Design review of the part shown in the three views and the two pictorial views. Dimensions are in mm from the part's minimum x, y and z. Coordinates: 2 decimals unless noted, no trailing zeros. Loops run counter-clockwise (first coordinate to the right, second up) from the corner with the lowest first, then second, coordinate; pieces in that order, holes last. Notation, with made-up numbers: M 65,59 L 103,59 A21 ccw 103,66 Z; hole C -9.5,-18.75 d9. An arc over 180 degrees is marked long. Use one line per item in the form item = value.
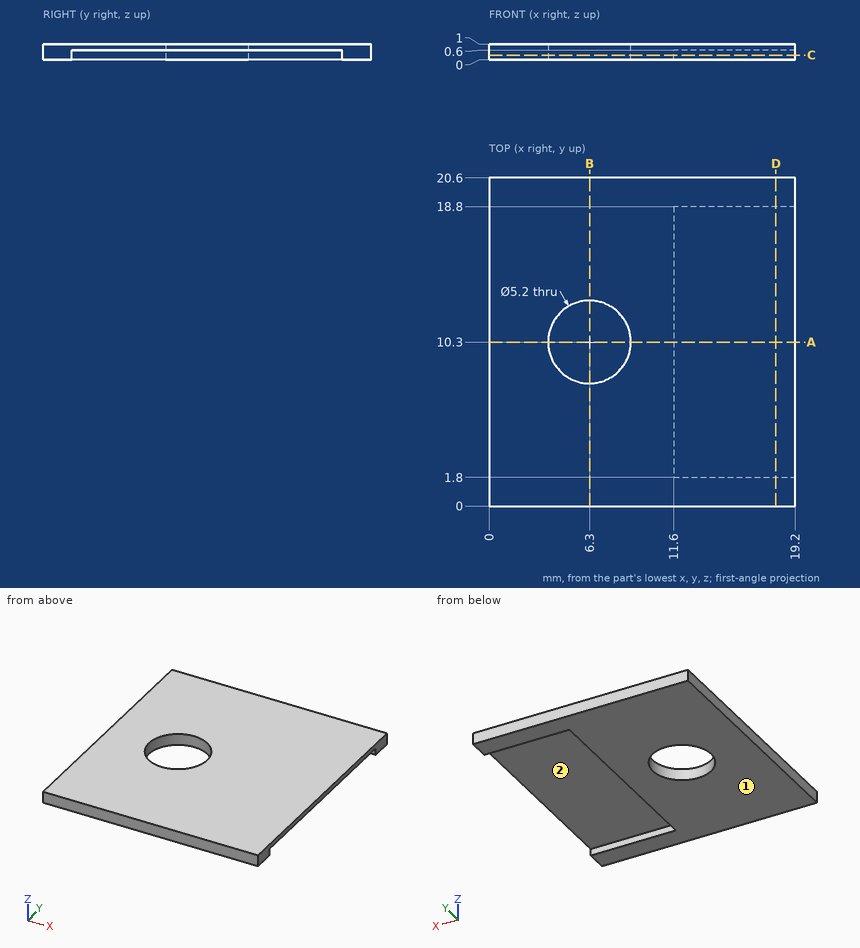
1. Add section D-D (x = 18). State the section outline as (y, z) points, then the cut area to 3 significant figures.
Response values:
outline = M 0,0 L 1.8,0 L 1.8,0.6 L 18.8,0.6 L 18.8,0 L 20.6,0 L 20.6,1 L 0,1 Z
area = 10.4 mm^2
2. Add section B-B (x = 6.3). State the section outline as (y, z) points.
Response values:
outline = M 0,0 L 7.7,0 L 7.7,1 L 0,1 Z; M 12.9,0 L 20.6,0 L 20.6,1 L 12.9,1 Z
3. Add section C-C (z = 0.3). State the section outline as (x, y) points, then the cut area to 3 significant figures.
Response values:
outline = M 0,0 L 19.2,0 L 19.2,1.8 L 11.6,1.8 L 11.6,18.8 L 19.2,18.8 L 19.2,20.6 L 0,20.6 Z; hole C 6.3,10.3 d5.2
area = 245 mm^2
4. Wall thickness on line 1 along Z through (x, y) = (16, 18); line 2 along X through (y, z) = (14.25, 0.4); line 3 along Y through (x, z) = (6.3, 0.55): over which ranges is each line inside the solid? List them lowest first. Write a range as from..to.
Response values:
line_1 = 0.6..1
line_2 = 0..11.6
line_3 = 0..7.7, 12.9..20.6
5. Add section A-A (y = 10.3). State the section outline as (x, z) points.
Response values:
outline = M 0,0 L 3.7,0 L 3.7,1 L 0,1 Z; M 8.9,0 L 11.6,0 L 11.6,0.6 L 19.2,0.6 L 19.2,1 L 8.9,1 Z
6. Insertion check: P1, Ø2.5, axis at x = 15, y = 7, coming from the -Z side. The pin has a flat end and moves straight along its axis. Give the tip position at first contact, or say it passes through.
Response values:
P1 = 0.6
7. The part is to be moulded in two halves that separate along Y. For the marked faces 1 and 2, say which applies: pulls with the +Y half, pulls with the -Y half, needs draft (parallel to the pull), parting line crosses it, or undercut.
Response values:
face_1 = needs draft
face_2 = undercut
